Print and shaded views of the part. All mm, measured from the part's lowest x, y and z. A direction names the side the tool comes from. Coordinates: 2 decimals unless noted, no trailing zeros. Order: outer loops, then holes, each group sorted by start corner. A loop starts at its lowest first (then second) coordinate and runs counter-clockwise, first axis right, second up. Notation, with made-up numbers: M -34,-25.75 L -15,-25.75 A21 ccw -15,11.25 Z; hole C 82.5,88 d3. An arc over 180 degrees is marked long. One line per item, written item: value.
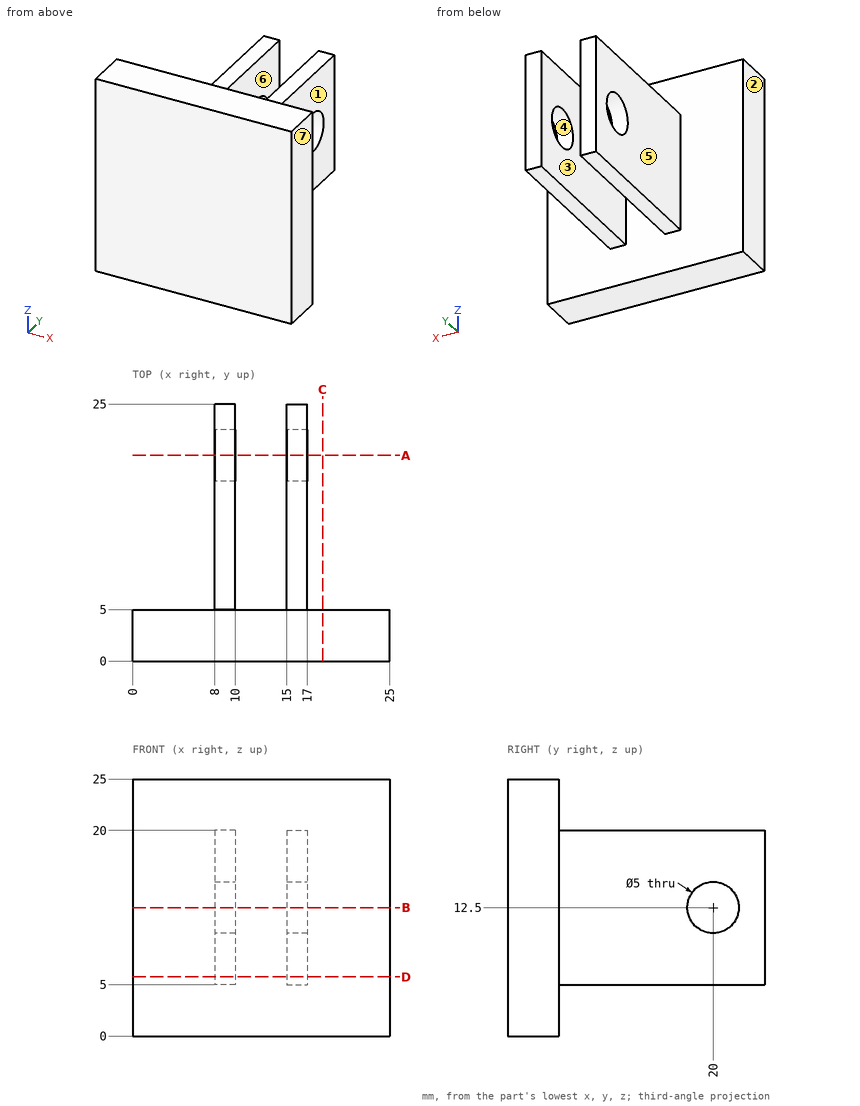
Q1. Slice it at A-A (y = 20). List the corners of the cut face in (x, z), plus the area to 3 significant figures.
Recorded:
outline: M 8,5 L 10,5 L 10,10 L 8,10 Z; M 8,15 L 10,15 L 10,20 L 8,20 Z; M 15,5 L 17,5 L 17,10 L 15,10 Z; M 15,15 L 17,15 L 17,20 L 15,20 Z
area: 40.0 mm^2
Q2. Which spindle directions (+Z, -Z, +X, -X, +Y, -Y) get a long thin tool onto all of the face, cutting with end or side? Do the marked faces 1, 2 and 3. Say none if no direction does.
Recorded:
face 1: +Z, -Z, +X, +Y
face 2: +Z, -Z, -X, +Y, -Y
face 3: +Z, -Z, +Y
Q3. Slice it at C-C (x = 18.5). List the corners of the cut face in (y, z).
Recorded:
outline: M 0,0 L 5,0 L 5,25 L 0,25 Z
Q4. Slice it at B-B (z = 12.5). List the corners of the cut face in (x, y).
Recorded:
outline: M 0,0 L 25,0 L 25,5 L 17,5 L 17,17.5 L 15,17.5 L 15,5 L 10,5 L 10,17.5 L 8,17.5 L 8,5 L 0,5 Z; M 8,22.5 L 10,22.5 L 10,25 L 8,25 Z; M 15,22.5 L 17,22.5 L 17,25 L 15,25 Z
Q5. Slice it at D-D (z = 5.75). List the corners of the cut face in (x, y), plus the area to 3 significant figures.
Recorded:
outline: M 0,0 L 25,0 L 25,5 L 17,5 L 17,25 L 15,25 L 15,5 L 10,5 L 10,25 L 8,25 L 8,5 L 0,5 Z
area: 205 mm^2
Q6. Pin check, flat tips, straight feed: pin 1 Ø1.6 at (x, y) = (15.5, 11.5) entering from -Z; pin 2 Ø8 at (x, y) = (3.5, 11.5) entering from -Z; pin 3 Ø2 at (x, y) = (8.5, 19.5) entering from +Z; pin 4 Ø8 at (y, z) = (11, 19) entering from -X. Stop position of each tip, or through.
Recorded:
pin 1: stops at z = 5
pin 2: passes through
pin 3: stops at z = 20
pin 4: stops at x = 8
Q7. Mould opens along X. For the marked faces 4, 5, 6 and 7 say: released by +X, released by -X, zero draft, split by the parting line, or undercut.
Recorded:
face 4: zero draft
face 5: released by -X
face 6: undercut
face 7: released by +X
Q8. Drill centre lines: line 1 along Y through (x, z) = (15.85, 12.5); line 2 along X through (y, z) = (18, 15); line 3 along Y through (x, z) = (9.5, 2.5). Where is each one in solid material? Low to high.
Recorded:
line 1: y = 0 to 17.5, 22.5 to 25
line 2: x = 8 to 10, 15 to 17
line 3: y = 0 to 5
